Model file for the job. Use its own axes, mm. A direction names the side the tool comes from. Round coordinates to 2 decimals unless told otherwise and drop trailing zeros. Order: outer loops, then holes, each group sorted by start corner. A loop starts at its lowest first (then second) coordinate and runs counter-clockwise, first axis right, second up. Notation, with made-up numbers: M 40.25,-16 L 91.25,-16 A18 ccw 91.25,12 Z; hole C 35,-32.5 d1. An arc over 180 degrees is marked long. Return JSON: item names as keys, results as strings. Group by question number.
Item 1: Which spindle directions (+Z, -Z, +X, -X, +Y, -Y) get a long thin tool onto all of the face, cutting with end or side? Do faces 4 (the face through (17.2, 143.8, -1)), 5 (the face through (11, 81, -2)), 6 (the face through (7.94, 83.18, 29.43)), 7 (the face through (1.8, 165, -13.8)). Say none if no direction does.
Item 2: Slice it at A-A on y = 117.5. Write the cut outline in (x, z).
Item 3: Slice it at C-C on z = -22.5. Write the cut outline in (x, y).
Item 4: Slice it at B-B on x = 15.75. Write the cut outline in (y, z).
Item 5: Slice it at D-D on y = 28. Write the cut outline in (x, z).
Item 6: Pull direction X, two halves, no side cores. Call faces 1 (the face through (6.8, 26.3, -1)), 2 (the face through (11, 81, 0)), 3 (the face through (0, 81, -20)): pulls with the +X half, pulls with the -X half, needs draft (parallel to the pull), parting line crosses it, or undercut.
Item 7: Pin check, flat tips, straight feed: pin 1 Ø9 at (x, y) = (12.5, 118) entering from -Z; pin 2 Ø8 at (x, z) = (5.5, -22.5) entering from -Y; pin 3 Ø10 at (x, y) = (3, 104) entering from +Z; pin 4 Ø10 at (x, z) = (8, -31.5) entering from +Y. Stop position of each tip, or through.
Item 8: Probe line 1 along Z through (x, y) = (6, 53); line 2 along X through (y, z) = (36, -3); line 3 along Y through (x, z) = (9, 4). List the from-to ranges inside material, lowest first.
from build123d import *

# Parameters (mm, degrees)
BOSS_EXTRUDE1_DEPTH = 165
CUT_EXTRUDE1_DEPTH  = 132
SKETCH5_R           = 3
SKETCH6_W           = 26
SKETCH6_H           = 12
CUT_EXTRUDE2_DEPTH  = 132
FILLET1_R           = 1
FILLET2_R           = 0.5


with BuildPart() as part:
    # Sketch1 → Boss-Extrude1 (new body)
    with BuildSketch(Plane(origin=(0, 0, 0), x_dir=(1, 0, 0), z_dir=(0, 1, 0))):
        Polygon((0, 0), (0, 40), (2, 40), (2, 2), (20.3, 2), (20.3, 0), align=None)
    extrude(amount=BOSS_EXTRUDE1_DEPTH)

    # Sketch2 → Cut-Extrude1 (cut)
    with BuildSketch(Plane.XY):
        with BuildLine():
            Line((13, 139.545), (11, 139.545))
            ThreePointArc((11, 139.545), (6.8, 143.745), (11, 147.945))
            Line((11, 147.945), (13, 147.945))
            ThreePointArc((13, 147.945), (17.2, 143.745), (13, 139.545))
        make_face()
        with BuildLine():
            Line((13, 30.455), (11, 30.455))
            ThreePointArc((11, 30.455), (6.8, 26.255), (11, 22.055))
            Line((11, 22.055), (13, 22.055))
            ThreePointArc((13, 22.055), (17.2, 26.255), (13, 30.455))
        make_face()
    extrude(amount=-CUT_EXTRUDE1_DEPTH, mode=Mode.SUBTRACT)

    # Sweep1: sweep along a path in Sketch4
    with BuildLine(Plane(origin=(10.15, 0, 0), x_dir=(0, 0, -1), z_dir=(1, 0, 0))) as sweep1_path:
        Line((0, 128.745), (-22.4, 128.745))
        ThreePointArc((-22.4, 128.745), (-25.935533906, 127.280533906), (-27.4, 123.745))
        Line((-27.4, 123.745), (-27.4, 43.745))
        ThreePointArc((-27.4, 43.745), (-25.935533906, 40.209466094), (-22.4, 38.745))
        Line((-22.4, 38.745), (0, 38.745))
    # Sketch5 → Sweep1 (sweep)
    with BuildSketch(Plane.XY):
        with Locations((10.15, 128.745)):
            Circle(SKETCH5_R)
    sweep(path=sweep1_path.line)

    # Sketch6 → Cut-Extrude2 (cut)
    with BuildSketch(Plane(origin=(2, 0, 0), x_dir=(0, 0, -1), z_dir=(1, 0, 0))):
        with Locations((27, 6)):
            Rectangle(SKETCH6_W, SKETCH6_H)
    extrude(amount=-CUT_EXTRUDE2_DEPTH, mode=Mode.SUBTRACT)

    # Fillet1
    fillet1_edges = [part.edges().sort_by_distance(p)[0] for p in [
        (0, 82.5, 0),
        (1, 165, -40),
        (1, 0, -14),
        (20.3, 165, -1),
        (1, 12, -14),
        (1, 12, -40),
    ]]
    fillet(fillet1_edges, radius=FILLET1_R)

    # Fillet2
    fillet2_edges = [part.edges().sort_by_distance(p)[0] for p in [
        (2, 82.5, -2),
    ]]
    fillet(fillet2_edges, radius=FILLET2_R)


solid = part.part
Output values:
{
 "1": {"face 4": "+Z, -Z", "face 5": "-Z, +X, +Y, -Y", "face 6": "none", "face 7": "+Z, -Z, +X, -X, +Y"},
 "2": {"outline": "M 0,-40 L 2,-40 L 2,-2.5 A0.5 cw 2.5,-2 L 20.3,-2 L 20.3,0 L 1,0 A1 ccw 0,-1 Z; C 10.15,27.4 d6"},
 "3": {"outline": "M 0,12 L 2,12 L 2,165 L 0,165 Z"},
 "4": {"outline": "M 0,-2 L 23.08,-2 L 23.08,0 L 0,0 Z; M 29.43,-2 L 140.57,-2 L 140.57,0 L 29.43,0 Z; M 146.92,-2 L 165,-2 L 165,0 L 146.92,0 Z"},
 "5": {"outline": "M 0,-40 L 2,-40 L 2,-2.5 A0.5 cw 2.5,-2 L 7.18,-2 L 7.18,0 L 1,0 A1 ccw 0,-1 Z; M 16.82,-2 L 20.3,-2 L 20.3,0 L 16.82,0 Z"},
 "6": {"face 1": "undercut", "face 2": "needs draft", "face 3": "pulls with the -X half"},
 "7": {"pin 1": "z = -2", "pin 2": "y = 12", "pin 3": "z = 29.49", "pin 4": "through"},
 "8": {"line 1": "-2 to 0", "line 2": "0 to 2", "line 3": "35.97 to 41.52, 125.97 to 131.52"}
}
